```python
from build123d import *

# Parameters (mm, degrees)
CUT_EXTRUDE1_START = -22
SKETCH2_R          = 2.1
CUT_EXTRUDE1_DEPTH = 22
CUT_EXTRUDE2_REACH = 86.691
SKETCH3_R          = 6


with BuildPart() as part:
    # Sketch1 → Revolve1 (revolve)
    with BuildSketch(Plane(origin=(0, 0, 0), x_dir=(0, 1, 0), z_dir=(0, 0, 1)), mode=Mode.PRIVATE) as revolve1_sk:
        Polygon((0, 0), (22, 0), (22, 26), (17, 26), (17, 36), (22, 48), (22, 70), (0, 70), align=None)
    revolve(revolve1_sk.sketch.rotate(Axis((-70, 0, 0), (1, 0, 0)), 180), axis=Axis((-70, 0, 0), (1, 0, 0)))

    # Sketch2 → Cut-Extrude1 (cut)
    with BuildSketch(Plane.YZ.offset(CUT_EXTRUDE1_START)):
        with Locations(Location((-11.5, 11.5, 0), (0, 0, 270))):
            Circle(SKETCH2_R)
        with Locations(Location((11.5, 11.5, 0), (0, 0, 270))):
            Circle(SKETCH2_R)
        with Locations(Location((11.5, -11.5, 0), (0, 0, 270))):
            Circle(SKETCH2_R)
        with Locations(Location((-11.5, -11.5, 0), (0, 0, 270))):
            Circle(SKETCH2_R)
        with BuildLine():
            Line((-8.5, 20.291623888), (8.5, 20.291623888))
            ThreePointArc((8.5, 20.291623888), (0, 22), (-8.5, 20.291623888))
        make_face()
        with BuildLine():
            Line((20.291623888, 8.5), (20.291623888, -8.5))
            ThreePointArc((20.291623888, -8.5), (22, 0), (20.291623888, 8.5))
        make_face()
        with BuildLine():
            Line((8.5, -20.291623888), (-8.5, -20.291623888))
            ThreePointArc((-8.5, -20.291623888), (0, -22), (8.5, -20.291623888))
        make_face()
        with BuildLine():
            Line((-20.291623888, -8.5), (-20.291623888, 8.5))
            ThreePointArc((-20.291623888, 8.5), (-22, 0), (-20.291623888, -8.5))
        make_face()
    extrude(amount=CUT_EXTRUDE1_DEPTH, mode=Mode.SUBTRACT)

    # Sketch3 → Cut-Extrude2 (cut, up to next)
    with BuildSketch(Plane(origin=(0, 20.291623888, 0), x_dir=(-1, 0, 0), z_dir=(0, 1, 0)), mode=Mode.PRIVATE) as cut_extrude2_sk1:
        with Locations(Location((13, 0, 0), (0, 0, 90))):
            Circle(SKETCH3_R)
    cut_extrude2_tool1 = extrude(cut_extrude2_sk1.sketch, amount=-CUT_EXTRUDE2_REACH, mode=Mode.PRIVATE) & part.part
    add(cut_extrude2_tool1.solids().sort_by_distance((-13, 20.291624, 0))[0], mode=Mode.SUBTRACT)


solid = part.part
```
For this review, take the finished solid that the model builds, in its own axes (mm). A direction names the side the tool comes from. Round coordinates to 2 decimals unless told otherwise and drop trailing zeros. Write each loop counter-clockwise with the first axis right and the second up, starting at its lowest first coordinate (ties: lowest second). Pieces come first, ordered by that corner, then holes. Notation, with made-up numbers: (88.5, 80.25) - (130.5, 80.25) arc R6 ccw to (130.5, 87.25) - close; hole circle Ø6 at (-24, 57.5). An arc over 180 degrees is marked (long way). Use CSV: the item, a comma, the result in double quotes.
1) Add section C-C on x = -4.5. Write out the cut boundary in (y, z).
Conclusion:
outline,"(-20.29, -8.5) arc R22 ccw to (-8.5, -20.29) - (8.5, -20.29) arc R22 ccw to (20.29, -8.5) - (20.29, 8.5) arc R22 ccw to (8.5, 20.29) - (-8.5, 20.29) arc R22 ccw to (-20.29, 8.5) - close; hole circle Ø4.2 at (-11.5, -11.5); hole circle Ø4.2 at (-11.5, 11.5); hole circle Ø4.2 at (11.5, -11.5); hole circle Ø4.2 at (11.5, 11.5)"
2) Add section B-B on y = 0. Write out the cut boundary in (x, z), and give its area (3 significant figures).
Conclusion:
outline,"(-70, -22) - (-48, -22) - (-36, -17) - (-26, -17) - (-26, -22) - (-22, -22) - (-22, -20.29) - (0, -20.29) - (0, 20.29) - (-22, 20.29) - (-22, 22) - (-26, 22) - (-26, 17) - (-36, 17) - (-48, 22) - (-70, 22) - close; hole circle Ø12 at (-13, 0)"
area,"2,730 mm^2"
3) Add section D-D on x = -60. Write out the cut boundary in (y, z), and give its area (3 significant figures).
Conclusion:
outline,"circle Ø44 at (0, 0)"
area,"1,520 mm^2"
4) Wall thickness on line 1 along Y through (x, z) = (-16, -11.5) (3 decimals); line 2 along Y through (x, z) = (-16, -11); line 3 along Z through (x, y) = (-9, -11): over which ranges is each line inside the solid? List them lowest first. Write a range as from..to.
Conclusion:
line 1,"y = -18.755..-13.6, -9.4..9.4, 13.6..18.755"
line 2,"y = -19.05..-13.54, -9.46..9.46, 13.54..19.05"
line 3,"z = -19.05..-13.54, -9.46..-4.47, 4.47..9.46, 13.54..19.05"
5) Add section A-A on x = -13. Write out the cut boundary in (y, z).
Conclusion:
outline,"(-20.29, -8.5) arc R22 ccw to (-8.5, -20.29) - (8.5, -20.29) arc R22 ccw to (20.29, -8.5) - (20.29, -6) - (-20.29, -6) - close; (-20.29, 6) - (20.29, 6) - (20.29, 8.5) arc R22 ccw to (8.5, 20.29) - (-8.5, 20.29) arc R22 ccw to (-20.29, 8.5) - close; hole circle Ø4.2 at (-11.5, -11.5); hole circle Ø4.2 at (-11.5, 11.5); hole circle Ø4.2 at (11.5, -11.5); hole circle Ø4.2 at (11.5, 11.5)"
6) For faces 1 (the conical face through (-36.751, -9.307, -14.598)), 2 (the flat face through (-6, -20.292, 0)), 3 (the flat face through (-22, 0, 21)), 4 (the cylindrical face through (-11.15, -11.41, -9.4)), list the 3-axis set-ups (+Z, -Z, +X, -X, +Y, -Y) from which the entire face can be reached by the end or side of a thin tool; tool diameter is ignored.
Conclusion:
face 1,"none"
face 2,"+Z, -Z, +X, -Y"
face 3,"+Z, +X, +Y, -Y"
face 4,"+X"
7) The part is to be moulded in two halves that separate along X. For faces 5 (the flat face through (-11, 0, 20.292)), 6 (the flat face through (-22, 12, -11)), 7 (the cylindrical face through (-7.05, 0.28, -0.78)), 8 (the cylindrical face through (-31.07, 2.213, -16.855)), say which applies: pulls with the +X half, pulls with the -X half, needs draft (parallel to the pull), parting line crosses it, or undercut.
Conclusion:
face 5,"needs draft"
face 6,"pulls with the +X half"
face 7,"undercut"
face 8,"undercut"
8) Clearance check with flat-ended pins moving along their axes: pin 1 Ø2 at (y, z) = (9.5, 0) entering from +X; pin 2 Ø4 at (y, z) = (-11.5, -11.5) entering from +X; pin 3 Ø8.5 at (x, y) = (-15.5, -2) entering from +Z; pin 4 Ø4 at (x, y) = (-54, -12) entering from -Z. State where each tip first meets the part, or that it passes through.
Conclusion:
pin 1,"stops at x = 0"
pin 2,"stops at x = -22"
pin 3,"stops at z = 20.29"
pin 4,"stops at z = -19.6"
